Input: part model. Units: mm. Frame: model coordinates. A direction names the side the tool comes from. Coordinates: 2 decimals unless noted, no trailing zeros. Order: outer loops, then holes, each group sorted by start corner. A loop starts at its lowest first (then second) coordinate and runs counter-clockwise, first axis right, second up. Notation, with made-up numbers: (58.5, 49) - (97.5, 49) arc R21 cw to (97.5, 87) - close; hole circle Ø9 at (79.5, 80). An arc over 180 degrees is marked (long way). Answer as CSV lines item,"result". Start each with the question number.
Item 1: Section C-C (x = 9.5). Output: boundary loops of the cut face in (y, z), and give its area (3 significant figures).
Item 2: Section D-D (x = 31). Output: boundary loops of the cut face in (y, z).
Item 3: Draft query along X for faces 1 (the cylindrical face through (35.21, 5.37, 27.57)), 2 (the flat face through (-12, 10.6, -24)), 3 (the cylindrical face through (32.05, 5.37, 21.95)), 4 (the flat face through (-23.889, 5, -1)). Return one class per face: +X half, -X half, draft (parallel to the pull), parting line (faces both ways), or undercut.
Item 4: Section B-B (z = -3.5). Output: boundary loops of the cut face in (x, y).
Item 5: Section A-A (x = -18). Output: boundary loops of the cut face in (y, z), and give its area (3 significant figures).
Item 6: First-contact query: pin 1 (8 mm diameter, centred on x = -8, z = 13, fed in from -Y); pin 2 (2 mm diameter, centred on x = -2.5, z = -7, fed in from +Y). Flat tips, straight axial feed; report the tip coordinate or a pass-through.
Item 7: Material intervals for line 1 along X through (y, z) = (2.5, -27); line 2 along X through (y, z) = (4, -28); line 3 along Z through (x, y) = (30, 9.5), sorted ascending.
Item 8: Access query for faces 5 (the flat face through (6, 10.5, -2)), 6 (the cylindrical face through (-23.033, 5.374, 27.524)), 7 (the flat face through (6, 0.1, -2)). Directions: +Z, -Z, +X, -X, +Y, -Y. A direction counts if a zero-diameter tool reaches every point of the face in a straight line with its end or side. Return the directions, or none.
from build123d import *

# Parameters (mm, degrees)
SKETCH1_W           = 60
SKETCH1_H           = 60
BOSS_EXTRUDE1_DEPTH = 10.6
FILLET1_R           = 3
SKETCH2_R           = 1.75
CUT_EXTRUDE1_DEPTH  = 11.6
CUT_EXTRUDE2_DEPTH  = 0.1
CUT_EXTRUDE3_START  = -10.6
CUT_EXTRUDE3_DEPTH  = 0.1


with BuildPart() as part:
    # Sketch1 → Boss-Extrude1 (new body)
    with BuildSketch(Plane(origin=(0, 0, 0), x_dir=(1, 0, 0), z_dir=(0, 1, 0))):
        with Locations((6.111111111, 1.574074074)):
            Rectangle(SKETCH1_W, SKETCH1_H)
    extrude(amount=BOSS_EXTRUDE1_DEPTH)

    # Fillet1
    fillet1_edges = [part.edges().sort_by_distance(p)[0] for p in [
        (-23.888888889, 5.3, -31.574074074),
        (36.111111111, 5.3, -31.574074074),
        (36.111111111, 5.3, 28.425925926),
        (-23.888888889, 5.3, 28.425925926),
    ]]
    fillet(fillet1_edges, radius=FILLET1_R)

    # Sketch2 → Cut-Extrude1 (cut, through all)
    with BuildSketch(Plane(origin=(0, 10.6, 0), x_dir=(1, 0, 0), z_dir=(0, 1, 0))):
        with Locations((-18.888888889, 26.574074074)):
            Circle(SKETCH2_R)
        with Locations((31.111111111, 26.574074074)):
            Circle(SKETCH2_R)
        with Locations((31.111111111, -23.425925926)):
            Circle(SKETCH2_R)
        with Locations((-18.888888889, -23.425925926)):
            Circle(SKETCH2_R)
    extrude(amount=-CUT_EXTRUDE1_DEPTH, mode=Mode.SUBTRACT)

    # Sketch3 → Cut-Extrude2 (cut)
    with BuildSketch(Plane(origin=(0, 10.6, 0), x_dir=(1, 0, 0), z_dir=(0, 1, 0))):
        with BuildLine():
            ThreePointArc((34.611111111, 1.574074074), (17.017588934, 27.904640751), (-14.041432153, 21.726617338))
            Line((-14.041432153, 21.726617338), (26.263654375, -18.57846919))
            ThreePointArc((26.263654375, -18.57846919), (32.441677788, -9.332403748), (34.611111111, 1.574074074))
        make_face()
        with BuildLine():
            Line((26.263654375, -18.57846919), (-14.041432153, 21.726617338))
            ThreePointArc((-14.041432153, 21.726617338), (-14.041432153, -18.57846919), (26.263654375, -18.57846919))
        make_face()
    extrude(amount=-CUT_EXTRUDE2_DEPTH, mode=Mode.SUBTRACT)

    # Sketch3<3> → Cut-Extrude3 (cut)
    with BuildSketch(Plane(origin=(0, 10.6, 0), x_dir=(1, 0, 0), z_dir=(0, 1, 0)).offset(CUT_EXTRUDE3_START)):
        with BuildLine():
            ThreePointArc((34.611111111, 1.574074074), (17.017588934, 27.904640751), (-14.041432153, 21.726617338))
            Line((-14.041432153, 21.726617338), (26.263654375, -18.57846919))
            ThreePointArc((26.263654375, -18.57846919), (32.441677788, -9.332403748), (34.611111111, 1.574074074))
        make_face()
        with BuildLine():
            Line((26.263654375, -18.57846919), (-14.041432153, 21.726617338))
            ThreePointArc((-14.041432153, 21.726617338), (-14.041432153, -18.57846919), (26.263654375, -18.57846919))
        make_face()
    extrude(amount=CUT_EXTRUDE3_DEPTH, mode=Mode.SUBTRACT)


solid = part.part
Determined:
1,outline,"(0, -31.57) - (10.6, -31.57) - (10.6, -29.87) - (10.5, -29.87) - (10.5, 26.72) - (10.6, 26.72) - (10.6, 28.43) - (0, 28.43) - (0, 26.72) - (0.1, 26.72) - (0.1, -29.87) - (0, -29.87) - close"
1,area,"625 mm^2"
2,outline,"(0, -31.57) - (10.6, -31.57) - (10.6, -28.32) - (0, -28.32) - close; (0, -24.83) - (10.6, -24.83) - (10.6, -15.46) - (10.5, -15.46) - (10.5, 12.31) - (10.6, 12.31) - (10.6, 21.68) - (0, 21.68) - (0, 12.31) - (0.1, 12.31) - (0.1, -15.46) - (0, -15.46) - close; (0, 25.17) - (10.6, 25.17) - (10.6, 28.43) - (0, 28.43) - close"
3,face 1,"+X half"
3,face 2,"draft"
3,face 3,"undercut"
3,face 4,"-X half"
4,outline,"(-23.89, 0) - (-22.32, 0) - (-22.32, 0.1) - (34.55, 0.1) - (34.55, 0) - (36.11, 0) - (36.11, 10.6) - (34.55, 10.6) - (34.55, 10.5) - (-22.32, 10.5) - (-22.32, 10.6) - (-23.89, 10.6) - close"
5,outline,"(0, -31.57) - (10.6, -31.57) - (10.6, -28.08) - (0, -28.08) - close; (0, -25.07) - (10.6, -25.07) - (10.6, -16.77) - (10.5, -16.77) - (10.5, 13.62) - (10.6, 13.62) - (10.6, 21.92) - (0, 21.92) - (0, 13.62) - (0.1, 13.62) - (0.1, -16.77) - (0, -16.77) - close; (0, 24.93) - (10.6, 24.93) - (10.6, 28.43) - (0, 28.43) - close"
5,area,"566 mm^2"
6,pin 1,"stops at y = 0.1"
6,pin 2,"stops at y = 10.5"
7,line 1,"x = -23.89 to -20.59, -17.19 to 29.41, 32.81 to 36.11"
7,line 2,"x = -23.89 to -19.9, -17.87 to 30.1, 32.13 to 36.11"
7,line 3,"z = -31.57 to -27.93, -25.22 to 22.07, 24.78 to 28.43"
8,face 5,"+Y"
8,face 6,"+Z, -X, +Y, -Y"
8,face 7,"-Y"
